Build history of the part. All positions in model axes, mm. A direction names the side the tool comes from. Round coordinates to 2 decimals unless told otherwise and drop trailing zeros. Write each loop counter-clockwise with the first axis right and the second up, starting at its lowest first coordinate (ties: lowest second). Pieces come first, ordered by that corner, then holes.
Item 1: Band-saw the part on B-B, the plane z = 13.75. Write the cut outline in (x, y), then the cut area to 3 significant figures.
Item 2: Drop flat-ended pins along their axis: pin 1 Ø3 at (x, y) = (0, -23.14) entering from +Z; pin 2 Ø1.6 at (y, z) = (-37, 3.5) entering from +X; pin 3 Ø1.6 at (x, z) = (4.5, 4) entering from +Y. Give the stop position or say it passes through.
Item 3: Band-saw the part on C-C, the plane x = 5.5. Write the cut outline in (y, z) (3 decimals).
Item 4: 3-axis set-ups, long thin cutter, end or side, ignore diameter. For faces 4 (the flat face through (3, -37, 7)), 5 (the flat face through (3, -10, 7)), 6 (the flat face through (-5, -7.355, 7)): which of +Z, -Z, +X, -X, +Y, -Y reach the whole face in a straight line?
Item 5: Mould opens along Y. For faces 1 (the flat face through (-3, -39.105, 7)), 2 (the flat face through (6, -12.605, 7)), 3 (the cylindrical face through (-0.39, -24.894, 7.43)) say: +Y half, -Y half, draft (parallel to the pull), parting line (faces both ways), or undercut.
Item 6: Wall check: probe 1 along Y at (x, z) = (0, 4); probe 2 along X at (y, z) = (-11, 1.75); probe 3 along X at (y, z) = (-23.5, 11.25). Give the ranges that are in metal, low to high.
Item 7: Band-saw the part on A-A, the plane x = 0. Write the cut outline in (y, z) (3 decimals), then the cut area to 3 significant figures.
```python
from build123d import *

# Parameters (mm, degrees)
SKETCH2_W           = 16.5
SKETCH2_H           = 31.75
BOSS_EXTRUDE1_DEPTH = 14.655
SKETCH5_W           = 5.25
SKETCH5_H           = 5.25
CUT_EXTRUDE2_DEPTH  = 15.655
SKETCH6_R           = 1.8
CUT_EXTRUDE3_DEPTH  = 15.655


with BuildPart() as part:
    # Sketch2 → Boss-Extrude1 (new body)
    with BuildSketch(Plane.XY):
        with Locations((0, -23.230249591)):
            Rectangle(SKETCH2_W, SKETCH2_H)
    extrude(amount=BOSS_EXTRUDE1_DEPTH)

    # Sketch5 → Cut-Extrude2 (cut, through all)
    with BuildSketch(Plane.XY.offset(14.655)):
        with Locations((5.625, -36.480249591)):
            Rectangle(SKETCH5_W, SKETCH5_H)
        with Locations((5.625, -9.980249591)):
            Rectangle(SKETCH5_W, SKETCH5_H)
    extrude(amount=-CUT_EXTRUDE2_DEPTH, mode=Mode.SUBTRACT)

    # Sketch6 → Cut-Extrude3 (cut, through all)
    with BuildSketch(Plane.XY.offset(14.655)):
        with Locations((0, -23.136715776)):
            Circle(SKETCH6_R)
        with Locations((0, -7.136715776)):
            Circle(SKETCH6_R)
    extrude(amount=-CUT_EXTRUDE3_DEPTH, mode=Mode.SUBTRACT)


solid = part.part
```
Results:
1. outline: (-8.25, -39.11) - (3, -39.11) - (3, -33.86) - (8.25, -33.86) - (8.25, -12.61) - (3, -12.61) - (3, -7.36) - (1.79, -7.36) arc R1.8 cw to (-1.79, -7.36) - (-8.25, -7.36) - close; hole circle Ø3.6 at (0, -23.14)
1. area: 454 mm2
2. pin 1: passes through
2. pin 2: stops at x = 3
2. pin 3: stops at y = -12.61
3. outline: (-33.855, 0) - (-12.605, 0) - (-12.605, 14.655) - (-33.855, 14.655) - close
4. face 4: +Z, -Z, +X, -Y
4. face 5: +Z, -Z, +X, +Y
4. face 6: +Z, -Z, +X, -X, +Y
5. face 1: -Y half
5. face 2: +Y half
5. face 3: undercut
6. probe 1: y = -39.11 to -24.94, -21.34 to -8.94
6. probe 2: x = -8.25 to 3
6. probe 3: x = -8.25 to -1.76, 1.76 to 8.25
7. outline: (-39.105, 0) - (-24.937, 0) - (-24.937, 14.655) - (-39.105, 14.655) - close; (-21.337, 0) - (-8.937, 0) - (-8.937, 14.655) - (-21.337, 14.655) - close
7. area: 389 mm2
